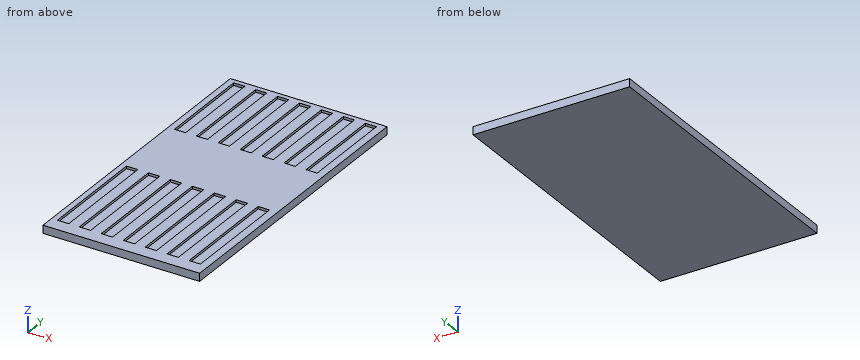
from build123d import *

# Parameters (mm, degrees)
F0_W     = 62.8318530718
F0_H     = 120
F1_DEPTH = 3.175
F2_W     = 4.4705853476
F2_H     = 38
F3_W     = 4.4705853476
F3_H     = 38
F3_W_2   = 4.565641284
F3_H_2   = 44.2867465317
F4_DEPTH = 1


# Not quite as in the source:
# - a length typed as a fraction of an inch, garbled in the dataset ("3 / 203.2 mm" for 3/8 in), is restored


with BuildPart() as f1:
    # F0 (on Top) → F1 (new body)
    with BuildSketch(Plane.XY):
        with Locations((-17.3296490684, 32.2412615943)):
            Rectangle(F0_W, F0_H)
    extrude(amount=F1_DEPTH)

    # F2 (on face) + F3 (on face) → F4 (cut)
    with BuildSketch(Plane.XY.offset(3.175)):
        with Locations((-26.3693033695, 71.3383685797)):
            Rectangle(F2_W, F2_H)
        with Locations((-43.9693033695, 71.3383685797)):
            Rectangle(F2_W, F2_H)
        with Locations((-35.1693033695, 71.3383685797)):
            Rectangle(F2_W, F2_H)
        with Locations((-8.7693033695, 71.3383685797)):
            Rectangle(F2_W, F2_H)
        with Locations((0.0306966305, 71.3383685797)):
            Rectangle(F2_W, F2_H)
        with Locations((8.8306966305, 71.3383685797)):
            Rectangle(F2_W, F2_H)
    with BuildSketch(Plane.XY.offset(3.175)):
        with Locations((-17.5693033695, 71.3383685797)):
            Rectangle(F3_W, F3_H)
        with Locations((-0.1788695753, -0.0753514469)):
            Rectangle(F3_W_2, F3_H_2)
        with Locations((-8.9788695753, -0.0753514469)):
            Rectangle(F3_W_2, F3_H_2)
        with Locations((-17.7788695753, -0.0753514469)):
            Rectangle(F3_W_2, F3_H_2)
        with Locations((-26.5788695753, -0.0753514469)):
            Rectangle(F3_W_2, F3_H_2)
        with Locations((-35.3788695753, -0.0753514469)):
            Rectangle(F3_W_2, F3_H_2)
        with Locations((-44.1788695753, -0.0753514469)):
            Rectangle(F3_W_2, F3_H_2)
        with Locations((8.6211304247, -0.0753514469)):
            Rectangle(F3_W_2, F3_H_2)
    extrude(amount=-F4_DEPTH, mode=Mode.SUBTRACT)


solid = f1.part
Geometry: final body of the model. Coordinates: model frame, mm. Give positions to 0.01 mm unless a question says otherwise; leave off trailing zeros. Write each loop counter-clockwise with the first axis right and the second up, starting at its lowest first coordinate (ties: lowest second). Pieces come first, ordered by that corner, then holes. Notation, with made-up numbers: (-25.75, -17) -> (-4.75, -17) arc R13 cw to (-4.75, 8) -> close; hole circle Ø4 at (-7.5, -9). An arc over 180 degrees is marked (long way). Answer as a JSON object with one key per item and string values.
1. Ray query, probe 1 along Y at (x, z) = (2, 2.7); probe 2 along Z at (x, y) = (-27, 60.5) (3 decimals); probe 3 along Y at (x, z) = (-33, 2.5). Return the intervals inside material, ascending. Write a range as from..to.
Ans:
{"probe 1": "y = -27.76..-22.22, 22.07..52.34, 90.34..92.24", "probe 2": "z = 0..2.175", "probe 3": "y = -27.76..52.34, 90.34..92.24"}
2. Contact query for a flat-ended pin moving along its axis: pin 1 (1.4 mm diameter, centred on x = -43, y = -1.5, fed in from +Z) (3 decimals). Output: stop coordinate, or through.
Ans:
{"pin 1": "stops at z = 2.175"}
3. Cut plane A-A on x = -25.5. Output: boundary loops of the cut face in (y, z) (3 decimals).
Ans:
{"outline": "(-27.759, 0) -> (92.241, 0) -> (92.241, 3.175) -> (90.338, 3.175) -> (90.338, 2.175) -> (52.338, 2.175) -> (52.338, 3.175) -> (22.068, 3.175) -> (22.068, 2.175) -> (-22.219, 2.175) -> (-22.219, 3.175) -> (-27.759, 3.175) -> close"}
